```python
from build123d import *

# Parameters (mm, degrees)
SKETCH_1_W          = 6
SKETCH_1_H          = 6
EXTRUDE_1_DEPTH     = 30
SKETCH_2_R          = 1.6
CUT_EXTRUDE_1_DEPTH = 5
CUT_EXTRUDE_START   = -30
SKETCH_2_2_R        = 1.6
CUT_EXTRUDE_2_DEPTH = 5
SKETCH_3_R          = 1.6
CUT_EXTRUDE_3_DEPTH = 7
SKETCH_4_R          = 1.6
CUT_EXTRUDE_4_DEPTH = 7


with BuildPart() as part:
    # 草图1 → 凸台-拉伸1 (new body)
    with BuildSketch(Plane.XY):
        with Locations((3, 3)):
            Rectangle(SKETCH_1_W, SKETCH_1_H)
    extrude(amount=EXTRUDE_1_DEPTH)

    # 草图2 → 切除-拉伸1 (cut)
    with BuildSketch(Plane.XY.offset(30)):
        with Locations((3, 3)):
            Circle(SKETCH_2_R)
    extrude(amount=-CUT_EXTRUDE_1_DEPTH, mode=Mode.SUBTRACT)

    # 草图2<2> → 切除-拉伸2 (cut)
    with BuildSketch(Plane.XY.offset(30).offset(CUT_EXTRUDE_START)):
        with Locations((3, 3)):
            Circle(SKETCH_2_2_R)
    extrude(amount=CUT_EXTRUDE_2_DEPTH, mode=Mode.SUBTRACT)

    # 草图3 → 切除-拉伸3 (cut)
    with BuildSketch(Plane(origin=(6, 0, 0), x_dir=(0, 0, -1), z_dir=(1, 0, 0))):
        with Locations((-22.5, 3)):
            Circle(SKETCH_3_R)
        with Locations((-12.5, 3)):
            Circle(SKETCH_3_R)
    extrude(amount=-CUT_EXTRUDE_3_DEPTH, mode=Mode.SUBTRACT)

    # 草图4 → 切除-拉伸4 (cut)
    with BuildSketch(Plane(origin=(0, 6, 0), x_dir=(1, 0, 0), z_dir=(0, 1, 0))):
        with Locations((3, -7.5)):
            Circle(SKETCH_4_R)
        with Locations((3, -17.5)):
            Circle(SKETCH_4_R)
    extrude(amount=-CUT_EXTRUDE_4_DEPTH, mode=Mode.SUBTRACT)


solid = part.part
```
The listing builds one solid part. Answer for the finished solid, in the listing's coordinates (mm). A direction names the side the tool comes from. Give positions to 0.01 mm unless a question says otherwise; leave off trailing zeros. Order: outer loops, then holes, each group sorted by start corner. A loop starts at its lowest first (then second) coordinate and runs counter-clockwise, first axis right, second up. Notation, with made-up numbers: (8, 69.25) -> (17, 69.25) arc R30 cw to (17, 94.25) -> close; hole circle Ø5 at (7, -31). An arc over 180 degrees is marked (long way). Answer as a JSON object with one key per item and string values. Group by question number.
Item 1: The part is cut by section B-B on z = 17.5. Write down the section's boundary in (x, y).
Item 2: Determine the mould class of faces 4 (the cylindrical face through (3.04, 3.07, 14.1)), 5 (the cylindrical face through (3.04, 1.58, 21.76)), 6 (the flat face through (3, 6, 15)), 7 (the cylindrical face through (2.792, 3.042, 15.914)) for opening direction Y: pulls with the +Y half, pulls with the -Y half, needs draft (parallel to the pull), parting line crosses it, or undercut.
Item 3: The part is cut by section A-A on y = 3. Write down the section's boundary in (x, z), and give its area (3 significant figures).
Item 4: A tool of negligible diameter and unlimited length cuts with its end or side. For faces 1 (the cylindrical face through (2.65, 1.44, 2.46)), 2 (the cylindrical face through (2.65, 1.44, 27.54)), 3 (the flat face through (6, 3, 15)), from which of +Z, -Z, +X, -X, +Y, -Y can it reach the whole face along a straight path? Write none if from no direction.
Item 5: The part is cut by section D-D on x = 1.05. Write down the section's boundary in (y, z).
Item 6: The part is cut by section C-C on x = 3.7. Write down the section's boundary in (y, z).
Item 7: Consider L1, parallel to Z at x = 4.7, y = 3.15; L2, parallel to X at y = 4.1, z = 17.5. Determine where each line is inside the solid, lowest interval first. Write a range as from..to.
Result set:
{
 "1": {"outline": "(0, 0) -> (1.4, 0) -> (1.4, 6) -> (0, 6) -> close; (4.6, 0) -> (6, 0) -> (6, 6) -> (4.6, 6) -> close"},
 "2": {"face 4": "undercut", "face 5": "undercut", "face 6": "pulls with the +Y half", "face 7": "needs draft"},
 "3": {"outline": "(0, 0) -> (1.4, 0) -> (1.4, 5) -> (4.6, 5) -> (4.6, 0) -> (6, 0) -> (6, 10.9) -> (0, 10.9) -> close; (0, 14.1) -> (6, 14.1) -> (6, 20.9) -> (0, 20.9) -> close; (0, 24.1) -> (6, 24.1) -> (6, 30) -> (4.6, 30) -> (4.6, 25) -> (1.4, 25) -> (1.4, 30) -> (0, 30) -> close; hole circle Ø3.2 at (3, 7.5); hole circle Ø3.2 at (3, 17.5)", "area": "93.5 mm²"},
 "4": {"face 1": "-Z", "face 2": "+Z", "face 3": "+Z, -Z, +X, +Y, -Y"},
 "5": {"outline": "(0, 0) -> (6, 0) -> (6, 30) -> (0, 30) -> close; hole circle Ø3.2 at (3, 12.5); hole circle Ø3.2 at (3, 22.5)"},
 "6": {"outline": "(0, 0) -> (1.56, 0) -> (1.56, 5) -> (4.44, 5) -> (4.44, 0) -> (6, 0) -> (6, 6.06) -> (0, 6.06) -> close; (0, 8.94) -> (6, 8.94) -> (6, 16.06) -> (0, 16.06) -> close; (0, 18.94) -> (6, 18.94) -> (6, 30) -> (4.44, 30) -> (4.44, 25) -> (1.56, 25) -> (1.56, 30) -> (0, 30) -> close; hole circle Ø3.2 at (3, 12.5); hole circle Ø3.2 at (3, 22.5)"},
 "7": {"L1": "0..10.91, 14.09..20.91, 24.09..30", "L2": "0..1.4, 4.6..6"}
}
